The drawing under review shows one solid part. Ordinate dimensions are in mm from its lowest x, y, z. Round coordinates to 2 decimals unless told otherwise and drop trailing zeros. Order: outer loops, then holes, each group sorted by start corner. A loop starts at its lowest first (then second) coordinate and runs counter-clockwise, first axis right, second up. Notation, with made-up numbers: M 4,-40 L 34,-40 A12 ccw 34,-29 Z; hole C -37,79.25 d8. An arc over 180 degrees is marked long. Use a Markdown table: item, result.
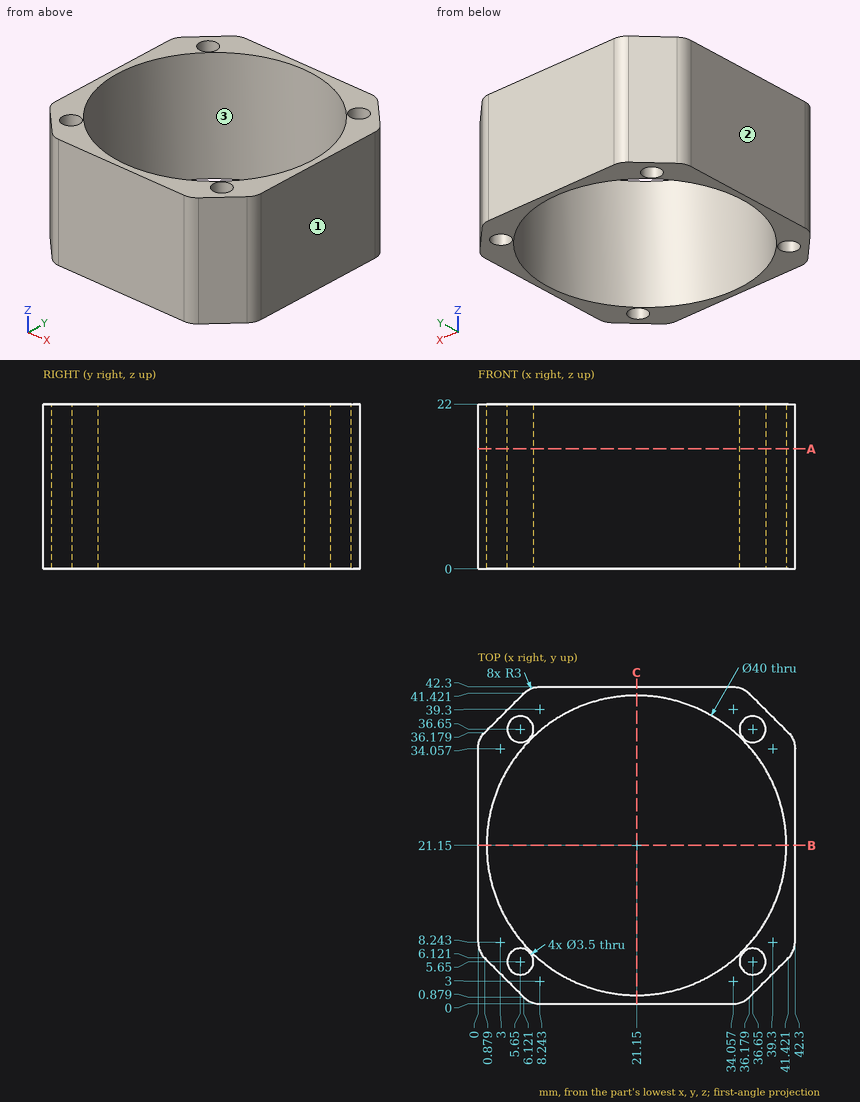
Q1. Clearance check with a flat-ended pin moving along its axis: pin 1 (3 mm diameter, centred on x = 4.5, z = 10.5, fed in from +Y). State where the tip first meets the part, or that it passes through.
Determined:
| item | result |
|---|---|
| pin 1 | stops at y = 41.3 |
Q2. Draft analysis for pull direction X (two halves, no side actions). For the marked faces 1, 2 and 3, state which applies: pulls with the +X half, pulls with the -X half, needs draft (parallel to the pull), parting line crosses it, or undercut.
Determined:
| item | result |
|---|---|
| face 1 | pulls with the +X half |
| face 2 | pulls with the -X half |
| face 3 | undercut |
Q3. Add section B-B (y = 21.15). Write out the cut boundary in (x, z).
Determined:
| item | result |
|---|---|
| outline | M 0,0 L 1.15,0 L 1.15,22 L 0,22 Z; M 41.15,0 L 42.3,0 L 42.3,22 L 41.15,22 Z |
Q4. Wall thickness on line 1 along Y through (x, z) = (21.5, 16); line 2 along X through (y, z) = (20.5, 8.75); line 3 along Y through (x, z) = (5.65, 8): over which ranges is each line inside the solid? List them lowest first. Write a range as [from, to].
Determined:
| item | result |
|---|---|
| line 1 | y = [0, 1.15], [41.15, 42.3] |
| line 2 | x = [0, 1.16], [41.14, 42.3] |
| line 3 | y = [1.35, 3.9], [7.4, 8.51], [33.79, 34.9], [38.4, 40.95] |
Q5. Add section A-A (z = 16). Write out the cut boundary in (x, y).
Determined:
| item | result |
|---|---|
| outline | M 0,8.24 A3 ccw 0.88,6.12 L 6.12,0.88 A3 ccw 8.24,0 L 34.06,0 A3 ccw 36.18,0.88 L 41.42,6.12 A3 ccw 42.3,8.24 L 42.3,34.06 A3 ccw 41.42,36.18 L 36.18,41.42 A3 ccw 34.06,42.3 L 8.24,42.3 A3 ccw 6.12,41.42 L 0.88,36.18 A3 ccw 0,34.06 Z; hole C 21.15,21.15 d40; hole C 5.65,5.65 d3.5; hole C 5.65,36.65 d3.5; hole C 36.65,5.65 d3.5; hole C 36.65,36.65 d3.5 |
